Part model, mm, in its own coordinate system. A direction names the side the tool comes from. Give positions to 0.01 mm unless a question says otherwise; leave off trailing zeros. Write each loop counter-clockwise with the first axis right and the second up, starting at its lowest first coordinate (ties: lowest second). Pieces come first, ordered by that corner, then holes. Notation, with made-up numbers: M 82,-22.5 L 99,-22.5 A31 cw 99,15.5 Z; hole C 85,80 d5. An arc over 180 degrees is marked long. Use a Markdown table: item, result.
```python
from build123d import *

# Parameters (mm, degrees)
ESQUISSE1_R        = 1.25
BOSS_EXTRU_1_DEPTH = 2
ESQUISSE2_R        = 1.5
BOSS_EXTRU_2_DEPTH = 6
ESQUISSE3_R        = 1.75
BOSS_EXTRU_3_DEPTH = 0.5


with BuildPart() as part:
    # Esquisse1 → Boss.-Extru.1 (new body)
    with BuildSketch(Plane.XY):
        with BuildLine():
            Line((9.75, -3), (-9.75, -3))
            ThreePointArc((-9.75, -3), (-12.503272584, -1.191423551), (-11.936875866, 2.053673282))
            Line((-11.936875866, 2.053673282), (-4.373751731, 10.107346563))
            ThreePointArc((-4.373751731, 10.107346563), (0, 12), (4.373751731, 10.107346563))
            Line((4.373751731, 10.107346563), (11.936875866, 2.053673282))
            ThreePointArc((11.936875866, 2.053673282), (12.503272584, -1.191423551), (9.75, -3))
        make_face()
        with Locations((0, 6)):
            Circle(ESQUISSE1_R, mode=Mode.SUBTRACT)
        with Locations((9.75, 0)):
            Circle(ESQUISSE1_R, mode=Mode.SUBTRACT)
        with Locations((-9.75, 0)):
            Circle(ESQUISSE1_R, mode=Mode.SUBTRACT)
    extrude(amount=BOSS_EXTRU_1_DEPTH)

    # Esquisse2 → Boss.-Extru.2 (add)
    with BuildSketch(Plane.XY.offset(2)):
        Circle(ESQUISSE2_R)
    extrude(amount=BOSS_EXTRU_2_DEPTH)

    # Esquisse3 → Boss.-Extru.3 (add)
    with BuildSketch(Plane.XY.offset(2)):
        Circle(ESQUISSE3_R)
    extrude(amount=BOSS_EXTRU_3_DEPTH)


solid = part.part
```
1. Cut at C-C, the plane y = 6. Give the cut face in (x, z), then the cut area to 3 significant figures.
Findings below:
| item | result |
|---|---|
| outline | M -8.23,0 L -1.25,0 L -1.25,2 L -8.23,2 Z; M 1.25,0 L 8.23,0 L 8.23,2 L 1.25,2 Z |
| area | 27.9 mm2 |
2. Tool access for faces 5 (the cylindrical face through (-1.5, 0.07, 5.21)), 6 (the flat face through (0, 3, 0)): list every direction of +Z, -Z, +X, -X, +Y, -Y with a clear straight run to the whole face (end or side of a thin tool).
Findings below:
| item | result |
|---|---|
| face 5 | +Z |
| face 6 | -Z, +X, -X, +Y, -Y |
3. Cut at B-B, the plane x = 0. Give the cut face in (y, z), then the cut area to 4 significant figures.
Findings below:
| item | result |
|---|---|
| outline | M -3,0 L 4.75,0 L 4.75,2 L 1.75,2 L 1.75,2.5 L 1.5,2.5 L 1.5,8 L -1.5,8 L -1.5,2.5 L -1.75,2.5 L -1.75,2 L -3,2 Z; M 7.25,0 L 12,0 L 12,2 L 7.25,2 Z |
| area | 43.25 mm2 |
4. Cut at D-D, the plane z = 6. Give the cut face in (x, y).
Findings below:
| item | result |
|---|---|
| outline | C 0,0 d3 |
5. Drop flat-ended pins along their axis: P1, Ø2, axis at x = -1, y = 7, coming from the +Z side; P2, Ø2, axis at y = -1, z = 7, coming from the +X side. Give the stop position or say it passes through.
Findings below:
| item | result |
|---|---|
| P1 | z = 2 |
| P2 | x = 1.5 |
6. Drill centre lines: L1, parallel to Z at x = -0.75, y = 8.5; L2, parallel to X at y = -0.25, z = 0.5; L3, parallel to Y at x = 9.75, z = 1.1. Where is each one in solid material? Low to high.
Findings below:
| item | result |
|---|---|
| L1 | 0 to 2 |
| L2 | -12.74 to -10.97, -8.53 to 8.53, 10.97 to 12.74 |
| L3 | -3 to -1.25, 1.25 to 4.38 |
7. Cut at A-A, the plane z = 0.5. Give the cut face in (x, y).
Findings below:
| item | result |
|---|---|
| outline | M -11.94,2.05 A3 ccw -9.75,-3 L 9.75,-3 A3 ccw 11.94,2.05 L 4.37,10.11 A6 ccw -4.37,10.11 Z; hole C -9.75,0 d2.5; hole C 0,6 d2.5; hole C 9.75,0 d2.5 |
8. Two-plate mould, pull along Y, no slides. Class faces 1 (the cylindrical face through (-12.5, -1.2, 1)), 2 (the flat face through (-8.21, 6.02, 0.99)), 3 (the cylindrical face through (-0.27, 4.78, 0.99)), 4 (the cylindrical face through (8.5, 0.05, 0.99)): released by +Y, released by -Y, zero draft, split by the parting line, or undercut.
Findings below:
| item | result |
|---|---|
| face 1 | split by the parting line |
| face 2 | released by +Y |
| face 3 | undercut |
| face 4 | undercut |
